Work out the finished part from the listing and answer in its coordinate system (mm). A direction names the side the tool comes from. Coordinates: 2 decimals unless noted, no trailing zeros. Order: outer loops, then holes, each group sorted by start corner. A loop starts at its lowest first (then second) coordinate and runs counter-clockwise, first axis right, second up. Notation, with made-up numbers: M 62,83.5 L 72,83.5 A9 cw 72,90.5 Z; hole C 18,54.5 d4. An arc over 180 degrees is marked long. Use a Markdown table: item, result.
from build123d import *

# Parameters (mm, degrees)
BOSS_EXTRUDE3_DEPTH = 10
SKETCH2_R           = 35
BOSS_EXTRUDE4_DEPTH = 15


with BuildPart() as part:
    # Sketch1 → Boss-Extrude3 (new body)
    with BuildSketch(Plane(origin=(0, 0, 0), x_dir=(1, 0, 0), z_dir=(0, 1, 0))):
        with BuildLine():
            Line((-7.5, 49.718353376), (-7.5, 99.718353376))
            ThreePointArc((-7.5, 99.718353376), (-12.371520282, 99.231776594), (-17.213387926, 98.507356457))
            ThreePointArc((-17.213387926, 98.507356457), (-38.890872965, 38.890872965), (-98.507356457, 17.213387926))
            ThreePointArc((-98.507356457, 17.213387926), (-99.231776594, 12.371520282), (-99.718353376, 7.5))
            Line((-99.718353376, 7.5), (-49.718353376, 7.5))
            ThreePointArc((-49.718353376, 7.5), (-42.218353376, 0), (-49.718353376, -7.5))
            Line((-49.718353376, -7.5), (-99.718353376, -7.5))
            ThreePointArc((-99.718353376, -7.5), (-99.231776594, -12.371520282), (-98.507356457, -17.213387926))
            ThreePointArc((-98.507356457, -17.213387926), (-38.890872965, -38.890872965), (-17.213387926, -98.507356457))
            ThreePointArc((-17.213387926, -98.507356457), (-12.371520282, -99.231776594), (-7.5, -99.718353376))
            Line((-7.5, -99.718353376), (-7.5, -49.718353376))
            ThreePointArc((-7.5, -49.718353376), (0, -42.218353376), (7.5, -49.718353376))
            Line((7.5, -49.718353376), (7.5, -99.718353376))
            ThreePointArc((7.5, -99.718353376), (12.371520282, -99.231776594), (17.213387926, -98.507356457))
            ThreePointArc((17.213387926, -98.507356457), (38.890872965, -38.890872965), (98.507356457, -17.213387926))
            ThreePointArc((98.507356457, -17.213387926), (99.231776594, -12.371520282), (99.718353376, -7.5))
            Line((99.718353376, -7.5), (49.718353376, -7.5))
            ThreePointArc((49.718353376, -7.5), (42.218353376, 0), (49.718353376, 7.5))
            Line((49.718353376, 7.5), (99.718353376, 7.5))
            ThreePointArc((99.718353376, 7.5), (99.231776594, 12.371520282), (98.507356457, 17.213387926))
            ThreePointArc((98.507356457, 17.213387926), (38.890872965, 38.890872965), (17.213387926, 98.507356457))
            ThreePointArc((17.213387926, 98.507356457), (12.371520282, 99.231776594), (7.5, 99.718353376))
            Line((7.5, 99.718353376), (7.5, 49.718353376))
            ThreePointArc((7.5, 49.718353376), (0, 42.218353376), (-7.5, 49.718353376))
        make_face()
    extrude(amount=BOSS_EXTRUDE3_DEPTH)

    # Sketch2 → Boss-Extrude4 (add)
    with BuildSketch(Plane(origin=(0, 10, 0), x_dir=(1, 0, 0), z_dir=(0, 1, 0))):
        with Locations(Location((0, 0, 0), (0, 0, 270))):
            Circle(SKETCH2_R)
        with BuildLine():
            Line((-5, 8.660254038), (-5, 30))
            Line((-5, 30), (5, 30))
            Line((5, 30), (5, 8.660254038))
            ThreePointArc((5, 8.660254038), (7.071067812, 7.071067812), (8.660254038, 5))
            Line((8.660254038, 5), (30, 5))
            Line((30, 5), (30, -5))
            Line((30, -5), (8.660254038, -5))
            ThreePointArc((8.660254038, -5), (7.071067812, -7.071067812), (5, -8.660254038))
            Line((5, -8.660254038), (5, -30))
            Line((5, -30), (-5, -30))
            Line((-5, -30), (-5, -8.660254038))
            ThreePointArc((-5, -8.660254038), (-7.071067812, -7.071067812), (-8.660254038, -5))
            Line((-8.660254038, -5), (-30, -5))
            Line((-30, -5), (-30, 5))
            Line((-30, 5), (-8.660254038, 5))
            ThreePointArc((-8.660254038, 5), (-7.071067812, 7.071067812), (-5, 8.660254038))
        make_face(mode=Mode.SUBTRACT)
    extrude(amount=BOSS_EXTRUDE4_DEPTH)


solid = part.part
(1) Given P1, Ø3, axis at x = -29, y = 14.5, coming from the +Z side; P2, Ø3, axis at y = 18.5, z = -1.5, coming from the +X side; P3, Ø12, axis at y = 17, z = -16, coming from the -X side; P4, Ø4, axis at x = -72.5, y = 13.5, coming from the +Z side, each flat-ended and moving along its own axis, determine where each tip first touches the part or whether it passes through.
Conclusion:
| item | result |
|---|---|
| P1 | z = 21.65 |
| P2 | x = 35 |
| P3 | x = -33.54 |
| P4 | through |
(2) A cutting plane is placed at D-D (x = 0). Determine the outline of the cut face in (y, z).
Conclusion:
| item | result |
|---|---|
| outline | M 0,-42.22 L 10,-42.22 L 10,-35 L 25,-35 L 25,-30 L 10,-30 L 10,30 L 25,30 L 25,35 L 10,35 L 10,42.22 L 0,42.22 Z |
(3) Straight lines are drawn through the part: L1, parallel to Y at x = -34, z = 35.5; L2, parallel to Z at x = 20, y = 22.5; L3, parallel to X at y = 23, z = 3. For each, find the intervals that lie inside material, in ascending order.
Conclusion:
| item | result |
|---|---|
| L1 | 0 to 10 |
| L2 | -28.72 to -5, 5 to 28.72 |
| L3 | -34.87 to -30, 30 to 34.87 |
(4) Which of the six approach directions +Z, -Z, +X, -X, +Y, -Y give full straight-line access (tool end or side, diameter ignored) to faces 1 (the flat face through (-30, 17, 0)), 2 (the flat face through (7.5, 5, 74)), 3 (the cylindrical face through (-42.22, 4.93, -0.16))?
Conclusion:
| item | result |
|---|---|
| face 1 | +Y |
| face 2 | +Z, +Y, -Y |
| face 3 | -X, +Y, -Y |
(5) A cutting plane is placed at A-A (y = 16.5). Determine the outline of the cut face in (x, z).
Conclusion:
| item | result |
|---|---|
| outline | C 0,0 d70; hole M -30,-5 L -8.66,-5 A10 ccw -5,-8.66 L -5,-30 L 5,-30 L 5,-8.66 A10 ccw 8.66,-5 L 30,-5 L 30,5 L 8.66,5 A10 ccw 5,8.66 L 5,30 L -5,30 L -5,8.66 A10 ccw -8.66,5 L -30,5 Z |
(6) A cutting plane is placed at B-B (z = 79.5). Determine the outline of the cut face in (x, y).
Conclusion:
| item | result |
|---|---|
| outline | M -17.96,0 L -7.5,0 L -7.5,10 L -17.96,10 Z; M 7.5,0 L 17.96,0 L 17.96,10 L 7.5,10 Z |
(7) A cutting plane is placed at C-C (y = 5). Determine the outline of the cut face in (x, z), then the cut area to 3 significant figures.
Conclusion:
| item | result |
|---|---|
| outline | M -99.72,-7.5 A100 ccw -98.51,-17.21 A75 cw -17.21,-98.51 A100 ccw -7.5,-99.72 L -7.5,-49.72 A7.5 cw 7.5,-49.72 L 7.5,-99.72 A100 ccw 17.21,-98.51 A75 cw 98.51,-17.21 A100 ccw 99.72,-7.5 L 49.72,-7.5 A7.5 cw 49.72,7.5 L 99.72,7.5 A100 ccw 98.51,17.21 A75 cw 17.21,98.51 A100 ccw 7.5,99.72 L 7.5,49.72 A7.5 cw -7.5,49.72 L -7.5,99.72 A100 ccw -17.21,98.51 A75 cw -98.51,17.21 A100 ccw -99.72,7.5 L -49.72,7.5 A7.5 cw -49.72,-7.5 Z |
| area | 13,800 mm2 |
(8) Determine the mould class of faces 4 (the cylindrical face through (-99.24, 4.93, 12.3)), 5 (the flat face through (-5, 17, -19)), 6 (the flat face through (-23, 10, -30)), 7 (the cylindrical face through (-0.16, 4.93, 42.22)) for opening direction X: pulls with the +X half, pulls with the -X half, needs draft (parallel to the pull), parting line crosses it, or undercut.
Conclusion:
| item | result |
|---|---|
| face 4 | pulls with the -X half |
| face 5 | undercut |
| face 6 | needs draft |
| face 7 | undercut |
